from build123d import *

# Parameters (mm, degrees)
EXTRUDE_1_DEPTH          = 120
SKETCH_1_4_R             = 20
EXTRUDE_1_2_DEPTH        = 20
CUT_EXTRUDE_1_DEPTH      = 270.814751265
CUT_EXTRUDE_1_DEPTH_BACK = 270.814751265
SKETCH_2_R               = 20


# Read off the part's stored shape, not the designer's step: 拉伸-薄壁1
with BuildPart() as part:
    # Extrude 1 outline → Extrude 1 (new body)
    with BuildSketch(Plane(origin=(0, 0, 0), x_dir=(1, 0, 0), z_dir=(0, 1, 0))):
        Polygon((-20, 0), (0, 0), (0, 80), (70, 80), (70, 0), (90, 0), (90, 100), (-20, 100), align=None)
    extrude(amount=EXTRUDE_1_DEPTH)

    # 草图1<4> → Extrude 1 2 (add)
    with BuildSketch(Plane(origin=(0, 0, 0), x_dir=(1, 0, 0), z_dir=(0, 1, 0))):
        with BuildLine():
            Line((90, 0), (185, 0))
            ThreePointArc((185, 0), (195.606601718, 4.393398282), (200, 15))
            Line((200, 15), (200, 85))
            ThreePointArc((200, 85), (195.606601718, 95.606601718), (185, 100))
            Line((185, 100), (90, 100))
            Line((90, 100), (90, 0))
        make_face()
        with Locations(Location((160, 40, 0), (0, 0, 270))):
            Circle(SKETCH_1_4_R, mode=Mode.SUBTRACT)
    extrude(amount=EXTRUDE_1_2_DEPTH)

    # 草图2 → 切除-拉伸1 (cut, two sides: drawn at the far end of the back side and taken through both)
    with BuildSketch(Plane.ZY.offset(20).offset(-CUT_EXTRUDE_1_DEPTH_BACK)):
        with Locations((-40, 80)):
            Circle(SKETCH_2_R)
    extrude(amount=CUT_EXTRUDE_1_DEPTH + CUT_EXTRUDE_1_DEPTH_BACK, mode=Mode.SUBTRACT)


solid = part.part
The model under review builds one solid part; all positions refer to its coordinate system, in mm. A direction names the side the tool comes from. Round coordinates to 2 decimals unless told otherwise and drop trailing zeros. Order: outer loops, then holes, each group sorted by start corner. A loop starts at its lowest first (then second) coordinate and runs counter-clockwise, first axis right, second up. Notation, with made-up numbers: (31.5, 19.5) - (35.5, 19.5) arc R4 cw to (35.5, 23.5) - close; hole circle Ø1 at (38.25, 21.25). An arc over 180 degrees is marked (long way). Use one line per item in the form item = value.
Q1. Add section B-B on z = -40. Give the boundary of the cut face in (x, y).
Response values:
outline = (-20, 0) - (0, 0) - (0, 60) - (-20, 60) - close; (-20, 100) - (0, 100) - (0, 120) - (-20, 120) - close; (70, 0) - (140, 0) - (140, 20) - (90, 20) - (90, 60) - (70, 60) - close; (70, 100) - (90, 100) - (90, 120) - (70, 120) - close; (180, 0) - (200, 0) - (200, 20) - (180, 20) - close
Q2. Mouldability with a two-part tool opening along Y and no side actions: class faces 4 (the flat face through (34, 120, -84)), 5 (the cylindrical face through (-9.86, 62.257, -30.771)), 6 (the cylindrical face through (195.49, 9.86, -4.28)) as pulls with the +Y half, pulls with the -Y half, needs draft (parallel to the pull), parting line crosses it, or undercut.
Response values:
face_4 = pulls with the +Y half
face_5 = undercut
face_6 = needs draft
Q3. Clearance check with flat-ended pins moving along their axes: P1, Ø6, axis at y = 53.5, z = -50, coming from the +X side; P2, Ø12, axis at y = 76, z = -27, coming from the +X side. State where each tip first meets the part, or that it passes through.
Response values:
P1 = 90
P2 = through
Q4. To check wall thickness, follow line 1 (X direction, y = 10.5, z = -40); line 2 (X direction, y = 113, z = -55.5); line 3 (Z direction, x = 83.75, y = 80). State the ranges of each line that lie inside material, in increasing order.
Response values:
line_1 = -20 to 0, 70 to 140, 180 to 200
line_2 = -20 to 0, 70 to 90
line_3 = -100 to -60, -20 to 0
Q5. Add section C-C on y = 11. Give the boundary of the cut face in (x, z).
Response values:
outline = (-20, -100) - (185, -100) arc R15 ccw to (200, -85) - (200, -15) arc R15 ccw to (185, 0) - (70, 0) - (70, -80) - (0, -80) - (0, 0) - (-20, 0) - close; hole circle Ø40 at (160, -40)
Q6. Add section A-A on y = 80. Give the boundary of the cut face in (x, z).
Response values:
outline = (-20, -100) - (90, -100) - (90, -60) - (70, -60) - (70, -80) - (0, -80) - (0, -60) - (-20, -60) - close; (-20, -20) - (0, -20) - (0, 0) - (-20, 0) - close; (70, -20) - (90, -20) - (90, 0) - (70, 0) - close
Q7. Add section D-D on z = -73.5. Give the boundary of the cut face in (x, y), then the cut area to 3 significant figures.
Response values:
outline = (-20, 0) - (0, 0) - (0, 120) - (-20, 120) - close; (70, 0) - (200, 0) - (200, 20) - (90, 20) - (90, 120) - (70, 120) - close
area = 7,000 mm^2
Q8. Tool access review of faces 1 (the flat face through (70, 59, -41)), 2 (the flat face through (144, 20, -62)), 3 (the flat face through (88, 32, 0)): name each direction out of +Z, -Z, +X, -X, +Y, -Y from which nothing blocks a thin tool from reaching the whole face with its end or side.
Response values:
face_1 = +Z, +Y, -Y
face_2 = +Z, -Z, +X, +Y
face_3 = +Z, +X, -X, +Y, -Y
